Autodesk Inventor part; units mm, degrees
ref_plane "YZ Plane" through (0, 0, 0) normal (1, 0, 0) x (0, 1, 0)
ref_plane "XZ Plane" through (0, 0, 0) normal (0, 1, 0) x (-1, 0, 0)
ref_plane "XY Plane" through (0, 0, 0) normal (0, 0, 1) x (1, 0, 0)
sketch "Sketch1" plane through (0, 0, 0) normal (0, 0, 1) x (1, 0, 0)
  line L0 (0.1582, 137.0969) -> (-25.2418, 137.0969)
  line L1 (-25.2418, 137.0969) -> (-25.2418, 162.4969)
  line L2 (-25.2418, 162.4969) -> (0.1582, 162.4969)
  line L3 (0.1582, 162.4969) -> (0.1582, 137.0969)
  point P0 (0, 0)
  dimension "d0" = 25.4
  dimension "d1" = 25.4
extrude "Extrusion1" add sketch "Sketch1" along normal blind 368.3
shell "Shell1" thickness 1.5875 removed faces 2 at (-8.3084, 145.5636, 0) at (-8.3084, 145.5636, 368.3)
properties part number "Frame_LowerConveyorBallSupport" material "Aluminum-6061"
Here's how the part is built. I have some questions about the finished solid (model axes, mm). A direction names the side the tool comes from. Round coordinates to 2 decimals unless told otherwise and drop trailing zeros. Order: outer loops, then holes, each group sorted by start corner. A loop starts at its lowest first (then second) coordinate and runs counter-clockwise, first axis right, second up. Notation, with made-up numbers: M -24.75,-6.75 L 13.25,-6.75 A22 cw 13.25,17.25 Z; hole C 12.5,61.5 d4. An arc over 180 degrees is marked long. One line per question, with ' | ' between items.
1) If we mould it in two halves opening along X, with no side actions, what happens to faces 3 (the face through (-12, 137.097, 182)), 4 (the face through (0.158, 150, 182)), 5 (the face through (-23.654, 150, 182))? For each: +X half, -X half, draft (parallel to the pull), parting line (faces both ways), or undercut.
Working result:
face 3: draft | face 4: +X half | face 5: undercut
2) I want a section at B-B, the plane y = 152.5. Write out the boundary of the cut face in (x, z), then the cut area to 3 significant figures.
Working result:
outline: M -25.24,0 L -23.65,0 L -23.65,368.3 L -25.24,368.3 Z; M -1.43,0 L 0.16,0 L 0.16,368.3 L -1.43,368.3 Z | area: 1,170 mm²
3) I need wall thicknesses on line 1 along Y through (x, z) = (-9.5, 210.5); line 2 along X through (y, z) = (160, 288). Which ranges of each line are inside material? Lowest first, please.
Working result:
line 1: 137.1 to 138.68, 160.91 to 162.5 | line 2: -25.24 to -23.65, -1.43 to 0.16
4) I want a section at C-C, the plane z = 174. Write out the boundary of the cut face in (x, y), then the cut area to 3 significant figures.
Working result:
outline: M -25.24,137.1 L 0.16,137.1 L 0.16,162.5 L -25.24,162.5 Z; hole M -23.65,138.68 L -1.43,138.68 L -1.43,160.91 L -23.65,160.91 Z | area: 151 mm²
5) For faces 1 (the face through (-1.429, 150, 182)), 2 (the face through (-13, 162.497, 182)), which set-ups out of +Z, -Z, +X, -X, +Y, -Y let a thin tool reach every point of the face, with its end or its side?
Working result:
face 1: +Z, -Z | face 2: +Z, -Z, +X, -X, +Y
6) For pin 1 Ø12 at (x, y) = (-18, 143.5) entering from -Z, with a flat end and sliding along its axis, tell me the tip position at first contact or that it passes through.
Working result:
pin 1: z = 0
7) I want a section at A-A, the plane x = -9.5. Write out the boundary of the cut face in (y, z).
Working result:
outline: M 137.1,0 L 138.68,0 L 138.68,368.3 L 137.1,368.3 Z; M 160.91,0 L 162.5,0 L 162.5,368.3 L 160.91,368.3 Z
